Build history of the part. All positions in model axes, mm. Give positions to 0.01 mm unless a question says otherwise; leave off trailing zeros. Order: outer loops, then holes, each group sorted by start corner. A loop starts at its lowest first (then second) coordinate and runs counter-clockwise, first axis right, second up. Notation, with made-up numbers: (89.5, 62.5) - (147.5, 62.5) arc R12 cw to (147.5, 84.5) - close; hole circle Ø5 at (1, 66.5). An arc over 180 degrees is marked (long way). One line per item, written item: value.
```python
from build123d import *

# Parameters (mm, degrees)
F1_DEPTH = 9.525
F2_D     = 6.096
F3_D     = 6.7564


with BuildPart() as f1:
    # F0 (on Top) → F1 (new body)
    with BuildSketch(Plane.XY):
        with BuildLine():
            Line((-101.6, 107.95), (-101.6, 0))
            ThreePointArc((-101.6, 0), (0, -101.6), (101.6, 0))
            Line((101.6, 0), (101.6, 107.95))
            Line((101.6, 107.95), (-101.6, 107.95))
        make_face()
    extrude(amount=F1_DEPTH)

    # F2 (through all)
    with Locations(Plane(origin=(0, 0, 0), x_dir=(1, 0, 0), z_dir=(0, 0, -1))):
        with Locations((-73.66, -34.9713074978), (73.66, -34.9713074978), (-55.245, 57.4458691038), (55.245, 57.4458691038)):
            Hole(F2_D / 2)

    # F3 (through all)
    with Locations(Plane(origin=(0, 0, 0), x_dir=(1, 0, 0), z_dir=(0, 0, -1))):
        with Locations((-48.075, -88.9), (0, -2.2420264777), (48.075, -88.9)):
            Hole(F3_D / 2)


solid = f1.part
```
(1) Pull direction Y, two halves, no side cores. Call faces 1 (the face through (1, 107.95, 5)), 2 (the face through (101.6, 53, 5)), 3 (the face through (72.3, 37.7, 4.8)): +Y half, -Y half, draft (parallel to the pull), parting line (faces both ways), or undercut.
Completed:
face 1: +Y half
face 2: draft
face 3: undercut
(2) Slice it at B-B, the plane y = 88.9. Give the cut face in (x, z) (3 decimals).
Completed:
outline: (-101.6, 0) - (-51.453, 0) - (-51.453, 9.525) - (-101.6, 9.525) - close; (-44.697, 0) - (44.697, 0) - (44.697, 9.525) - (-44.697, 9.525) - close; (51.453, 0) - (101.6, 0) - (101.6, 9.525) - (51.453, 9.525) - close
(3) Slice it at A-A, the plane x = 0. Give the cut face in (y, z) (3 decimals).
Completed:
outline: (-101.6, 0) - (-1.136, 0) - (-1.136, 9.525) - (-101.6, 9.525) - close; (5.62, 0) - (107.95, 0) - (107.95, 9.525) - (5.62, 9.525) - close
(4) Slice it at D-D, the plane x = -73.66. Give the cut face in (y, z) (3 decimals).
Completed:
outline: (-69.977, 0) - (31.923, 0) - (31.923, 9.525) - (-69.977, 9.525) - close; (38.019, 0) - (107.95, 0) - (107.95, 9.525) - (38.019, 9.525) - close
(5) Pin check, flat tips, straight feed: P1, Ø2, axis at x = -53.5, z = 4.5, coming from the -Y side; P2, Ø4, axis at y = -12.5, z = 1.5, coming from the -X side. Stop position of each tip, or through.
Completed:
P1: y = -86.98
P2: x = -101.06
(6) Slice it at C-C, the plane z = 5. Give the cut face in (x, y) (3 decimals).
Completed:
outline: (-101.6, 0) arc R101.6 ccw to (101.6, 0) - (101.6, 107.95) - (-101.6, 107.95) - close; hole circle Ø6.096 at (-73.66, 34.971); hole circle Ø6.096 at (-55.245, -57.446); hole circle Ø6.756 at (-48.075, 88.9); hole circle Ø6.756 at (0, 2.242); hole circle Ø6.756 at (48.075, 88.9); hole circle Ø6.096 at (55.245, -57.446); hole circle Ø6.096 at (73.66, 34.971)
(7) Drill centre lines: line 1 (X direction, y = 88.9, z = 3.5); line 2 (Y direction, x = 0, z = 6.5); line 3 (Y direction, x = -48.5, z = 4.75). Where is each one in solid material? Low to high.
Completed:
line 1: -101.6 to -51.45, -44.7 to 44.7, 51.45 to 101.6
line 2: -101.6 to -1.14, 5.62 to 107.95
line 3: -89.28 to 85.55, 92.25 to 107.95
